Autodesk Fusion 360 part; units mm, degrees
sketch "Sketch1" plane through (0, 0, 0) normal (0, 0, 1) x (1, 0, 0)
  line L0 (-10, 25) -> (-2.5, 25)
  line L1 (-2.5, 25) -> (-2.5, 20)
  arc A0 (-2.5, 20) -> (0, 17.5) centre (0, 20) ccw
  arc A1 (0, 17.5) -> (2.5, 20) centre (0, 20) ccw
  line L2 (2.5, 20) -> (2.5, 25)
  line L3 (2.5, 25) -> (10, 25)
  line L4 (0, 0) -> (0, 20) construction
  line L5 (0, 0) -> (10, 0) construction
  line L6 (-10, -25) -> (-2.5, -25)
  line L7 (-2.5, -25) -> (-2.5, -20)
  arc A2 (0, -17.5) -> (-2.5, -20) centre (0, -20) ccw
  arc A3 (2.5, -20) -> (0, -17.5) centre (0, -20) ccw
  line L8 (2.5, -20) -> (2.5, -25)
  line L9 (2.5, -25) -> (10, -25)
  line L10 (10, -25) -> (10, 25)
  line L11 (-10, -25) -> (-10, 25)
  line L12 (-10, 17.5) -> (10, 17.5) construction
  line L13 (-37.5, 25) -> (-30, 25)
  line L14 (-37.5, 20) -> (-37.5, 25)
  arc A4 (-40, 17.5) -> (-37.5, 20) centre (-40, 20) ccw
  arc A5 (-42.5, 20) -> (-40, 17.5) centre (-40, 20) ccw
  line L15 (-42.5, 25) -> (-42.5, 20)
  line L16 (-50, 25) -> (-42.5, 25)
  line L17 (-50, -25) -> (-50, 25)
  line L18 (-50, -25) -> (-42.5, -25)
  line L19 (-42.5, -25) -> (-42.5, -20)
  arc A6 (-40, -17.5) -> (-42.5, -20) centre (-40, -20) ccw
  arc A7 (-37.5, -20) -> (-40, -17.5) centre (-40, -20) ccw
  line L20 (-37.5, -20) -> (-37.5, -25)
  line L21 (-37.5, -25) -> (-30, -25)
  line L22 (-30, -25) -> (-30, 25)
  line L23 (-17.5, 25) -> (-10, 25)
  line L24 (-17.5, 20) -> (-17.5, 25)
  arc A8 (-20, 17.5) -> (-17.5, 20) centre (-20, 20) ccw
  arc A9 (-22.5, 20) -> (-20, 17.5) centre (-20, 20) ccw
  line L25 (-22.5, 25) -> (-22.5, 20)
  line L26 (-30, 25) -> (-22.5, 25)
  line L27 (-30, -25) -> (-30, 25)
  line L28 (-30, -25) -> (-22.5, -25)
  line L29 (-22.5, -25) -> (-22.5, -20)
  arc A10 (-20, -17.5) -> (-22.5, -20) centre (-20, -20) ccw
  arc A11 (-17.5, -20) -> (-20, -17.5) centre (-20, -20) ccw
  line L30 (-17.5, -20) -> (-17.5, -25)
  line L31 (-17.5, -25) -> (-10, -25)
  line L32 (-10, -25) -> (-10, 25)
  line L33 (22.5, 25) -> (30, 25)
  line L34 (22.5, 20) -> (22.5, 25)
  arc A12 (20, 17.5) -> (22.5, 20) centre (20, 20) ccw
  arc A13 (17.5, 20) -> (20, 17.5) centre (20, 20) ccw
  line L35 (17.5, 25) -> (17.5, 20)
  line L36 (10, 25) -> (17.5, 25)
  line L37 (10, -25) -> (10, 25)
  line L38 (10, -25) -> (17.5, -25)
  line L39 (17.5, -25) -> (17.5, -20)
  arc A14 (20, -17.5) -> (17.5, -20) centre (20, -20) ccw
  arc A15 (22.5, -20) -> (20, -17.5) centre (20, -20) ccw
  line L40 (22.5, -20) -> (22.5, -25)
  line L41 (22.5, -25) -> (30, -25)
  line L42 (30, -25) -> (30, 25)
  line L43 (42.5, 25) -> (50, 25)
  line L44 (42.5, 20) -> (42.5, 25)
  arc A16 (40, 17.5) -> (42.5, 20) centre (40, 20) ccw
  arc A17 (37.5, 20) -> (40, 17.5) centre (40, 20) ccw
  line L45 (37.5, 25) -> (37.5, 20)
  line L46 (30, 25) -> (37.5, 25)
  line L47 (30, -25) -> (30, 25)
  line L48 (30, -25) -> (37.5, -25)
  line L49 (37.5, -25) -> (37.5, -20)
  arc A18 (40, -17.5) -> (37.5, -20) centre (40, -20) ccw
  arc A19 (42.5, -20) -> (40, -17.5) centre (40, -20) ccw
  line L50 (42.5, -20) -> (42.5, -25)
  line L51 (42.5, -25) -> (50, -25)
  line L52 (50, -25) -> (50, 25)
  dimension "Notch_Radius" = 2.5
  dimension "Notch_Height" = 7.5
  dimension "Total_Height" = 50
  dimension "Repeat_Length" = 20
  dimension "Repeat_Spacing" = 20
  dimension "d8" = 0
extrude "Extrude1" add sketch "Sketch1" along normal mid plane 5
Check sheet for the modelled part. Datum: model origin and axes. Units: mm. A direction names the side the tool comes from. Round coordinates to 2 decimals unless told otherwise and drop trailing zeros. Loops run counter-clockwise (first coordinate to the right, second up) from the corner with the lowest first, then second, coordinate; pieces in that order, holes last. Notation, with made-up numbers: M -15,-26 L -10,-26 A25 cw -10,-6 Z; hole C 45,17.25 d5. An arc over 180 degrees is marked long. One line per item, written item: value.
(1) Access from +Z, -Z, +X, -X, +Y, -Y to the whole of each face (thin tool, end or side, straight path). Record for faces 4 (the face through (-17.5, 22, 0)), 5 (the face through (10, 25, 0)), 6 (the face through (-2.5, -23, 0)).
Computed values:
face 4: +Z, -Z, +Y
face 5: +Z, -Z, +X, -X, +Y
face 6: +Z, -Z, -Y
(2) Release check for a two-part mould opening along X. For faces 1 (the face through (50, 0, 0)), 2 (the face through (-39.9, 17.5, 0)), 3 (the face through (-10, 25, 0)) record: +X half, -X half, draft (parallel to the pull), parting line (faces both ways), or undercut.
Computed values:
face 1: +X half
face 2: undercut
face 3: draft
(3) Thickness scan on line 1 (X direction, y = -23, z = 0.85); line 2 (X direction, y = 18.5, z = 1.4); line 3 (Y direction, x = -2, z = -2). Record the ranges inside material, lowest first.
Computed values:
line 1: x = -50 to -42.5, -37.5 to -22.5, -17.5 to -2.5, 2.5 to 17.5, 22.5 to 37.5, 42.5 to 50
line 2: x = -50 to -42, -38 to -22, -18 to -2, 2 to 18, 22 to 38, 42 to 50
line 3: y = -18.5 to 18.5
(4) Sectioned sample at A-A, the plane x = 0. Record the cut outline in (y, z).
Computed values:
outline: M -17.5,-2.5 L 17.5,-2.5 L 17.5,2.5 L -17.5,2.5 Z
